The listing builds one solid part. Answer for the finished solid, in the listing's coordinates (mm). Face numbers are marked on the shaded views. A direction names the side the tool comes from. Round coordinates to 2 decimals unless told otherwise and drop trailing zeros. Loops run counter-clockwise (first coordinate to the right, second up) from the corner with the lowest first, then second, coordinate; pieces in that order, holes last. Notation, with made-up numbers: (70, -25.75) -> (112, -25.75) arc R18 cw to (112, 8.25) -> close; hole circle Ø2 at (57, 84). An arc over 180 degrees is marked (long way). Use a Markdown table: item, result. Add a question column.
Q1. Section D-D on y = 4.5 is taken. Give the vertices of the cut face in (x, z), then the cut area to 3 significant figures.
Q2. Given pin 1 Ø8 at (x, y) = (-5, 7) entering from +Z; pin 2 Ø1 at (y, z) = (10, 3.5) entering from +X; pin 3 Ø3 at (x, z) = (13.5, 6) entering from +Y; pin 4 Ø4 at (y, z) = (12.5, 6.5) entering from -X, each flat-ended and moving along its own axis, determine where each tip first touches the part or whether it passes through.
Q3. Section A-A on y = 2.25 is taken. Give the vertices of the cut face in (x, z).
Q4. Which of the six approach directions +Z, -Z, +X, -X, +Y, -Y give full straight-line access (tool end or side, diameter ignored) to the marked faces 4 and 5?
Q5. For a pull along X with two mould halves and no side action, classify the marked faces 1, 2 and 3 as released by +X, released by -X, zero draft, split by the parting line, or undercut.
Q6. Section C-C on x = 17 is taken. Give the vertices of the cut face in (y, z).
Q7. Consider line 1 (Z direction, x = 17, y = 1.95); line 2 (X direction, y = 2, z = 5); line 3 (X direction, y = 2.15, z = 5). Determine where each line is inside the solid, lowest interval first.
Q8. Section B-B on z = 5 is taken. Give the vertices of the cut face in (x, y).
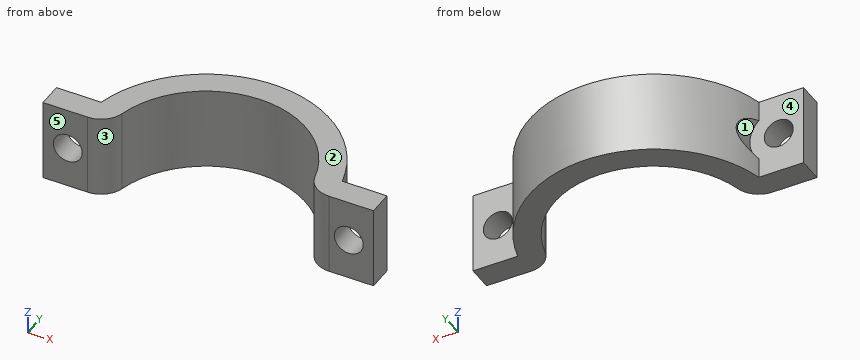
from build123d import *

# Parameters (mm, degrees)
BOSS_EXTRU_2_DEPTH      = 10
ESQUISSE3_R             = 1.75
ENL_V_MAT_EXTRU_2_DEPTH = 4
ESQUISSE4_R             = 3.5
ENL_V_MAT_EXTRU_3_DEPTH = 12.5


with BuildPart() as part:
    # Esquisse1 → Boss.-Extru.2 (new body)
    with BuildSketch(Plane.XY):
        with BuildLine():
            Line((-20, 0.5), (-14.585952146, 0.5))
            ThreePointArc((-14.585952146, 0.5), (-12.728534584, 1.144156202), (-11.668761717, 2.8))
            ThreePointArc((-11.668761717, 2.8), (0, 12), (11.668761717, 2.8))
            ThreePointArc((11.668761717, 2.8), (12.728534584, 1.144156202), (14.585952146, 0.5))
            Line((14.585952146, 0.5), (20, 0.5))
            Line((20, 0.5), (20, 3.5))
            Line((20, 3.5), (14.585952146, 3.5))
            ThreePointArc((14.585952146, 3.5), (0, 15), (-14.585952146, 3.5))
            Line((-14.585952146, 3.5), (-20, 3.5))
            Line((-20, 3.5), (-20, 0.5))
        make_face()
    extrude(amount=BOSS_EXTRU_2_DEPTH)

    # Esquisse3 → Enlèv. mat.-Extru.2 (cut, through all)
    with BuildSketch(Plane(origin=(0, 3.5, 0), x_dir=(1, 0, 0), z_dir=(0, 1, 0))):
        with Locations((-17, -5)):
            Circle(ESQUISSE3_R)
        with Locations((17, -5)):
            Circle(ESQUISSE3_R)
    extrude(amount=-ENL_V_MAT_EXTRU_2_DEPTH, mode=Mode.SUBTRACT)

    # Esquisse4 → Enlèv. mat.-Extru.3 (cut, through all)
    with BuildSketch(Plane(origin=(0, 3.5, 0), x_dir=(1, 0, 0), z_dir=(0, 1, 0))):
        with Locations((-17, -5)):
            Circle(ESQUISSE4_R)
        with Locations((17, -5)):
            Circle(ESQUISSE4_R)
    extrude(amount=ENL_V_MAT_EXTRU_3_DEPTH, mode=Mode.SUBTRACT)


solid = part.part
Checked values:
| question | item | result |
|---|---|---|
| 1 | outline | (-14.31, 0) -> (-11.12, 0) -> (-11.12, 10) -> (-14.31, 10) -> (-14.31, 7.24) arc R3.5 cw to (-14.31, 2.76) -> close; (11.12, 0) -> (14.31, 0) -> (14.31, 2.76) arc R3.5 cw to (14.31, 7.24) -> (14.31, 10) -> (11.12, 10) -> close |
| 1 | area | 58.7 mm2 |
| 2 | pin 1 | stops at z = 10 |
| 2 | pin 2 | stops at x = 11.61 |
| 2 | pin 3 | stops at y = 9 |
| 2 | pin 4 | stops at x = -10.71 |
| 3 | outline | (-20, 0) -> (-11.86, 0) -> (-11.86, 10) -> (-20, 10) -> close; (11.86, 0) -> (20, 0) -> (20, 10) -> (11.86, 10) -> close; hole circle Ø3.5 at (-17, 5); hole circle Ø3.5 at (17, 5) |
| 4 | face 4 | -X, +Y |
| 4 | face 5 | +Z, -Z, +X, -X, -Y |
| 5 | face 1 | released by -X |
| 5 | face 2 | zero draft |
| 5 | face 3 | undercut |
| 6 | outline | (0.5, 0) -> (3.5, 0) -> (3.5, 3.25) -> (0.5, 3.25) -> close; (0.5, 6.75) -> (3.5, 6.75) -> (3.5, 10) -> (0.5, 10) -> close |
| 7 | line 1 | z = 0 to 3.25, 6.75 to 10 |
| 7 | line 2 | x = -20 to -18.75, -15.25 to -11.99, 11.99 to 15.25, 18.75 to 20 |
| 7 | line 3 | x = -20 to -18.75, -15.25 to -11.91, 11.91 to 15.25, 18.75 to 20 |
| 8 | outline | (-20, 0.5) -> (-18.75, 0.5) -> (-18.75, 3.5) -> (-20, 3.5) -> close; (-15.25, 0.5) -> (-14.59, 0.5) arc R3 ccw to (-11.67, 2.8) arc R12 cw to (11.67, 2.8) arc R3 ccw to (14.59, 0.5) -> (15.25, 0.5) -> (15.25, 3.5) -> (13.5, 3.5) -> (13.5, 6.54) arc R15 ccw to (-13.5, 6.54) -> (-13.5, 3.5) -> (-15.25, 3.5) -> close; (18.75, 0.5) -> (20, 0.5) -> (20, 3.5) -> (18.75, 3.5) -> close |
